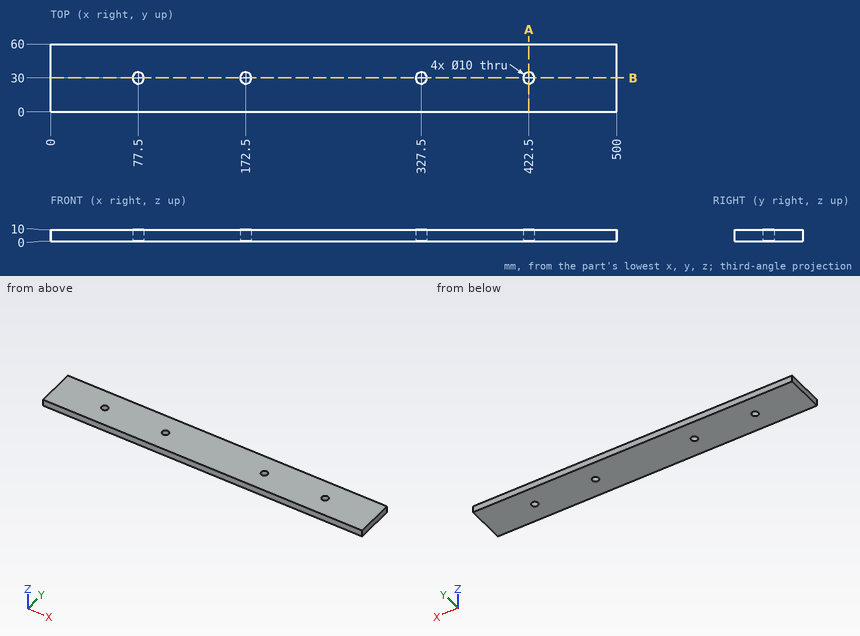
Job drawing, mm, ordinate dimensions from the low corner. One solid piece. Round coordinates to 2 decimals unless told otherwise and drop trailing zeros. Write each loop counter-clockwise with the first axis right and the second up, starting at its lowest first coordinate (ties: lowest second). Pieces come first, ordered by that corner, then holes.
1) Band-saw the part on B-B, the plane y = 30. List the corners of the cut face in (x, z), and give its area (3 significant figures).
2) Drill centre lines: probe 1 along Y at (x, z) = (422.5, 3.25); probe 2 along Y at (x, z) = (330.5, 6.5). Where is each one in solid material? Low to high.
3) Band-saw the part on A-A, the plane x = 422.5. List the corners of the cut face in (y, z).
Ans:
1. outline: (0, 0) - (72.5, 0) - (72.5, 10) - (0, 10) - close; (82.5, 0) - (167.5, 0) - (167.5, 10) - (82.5, 10) - close; (177.5, 0) - (322.5, 0) - (322.5, 10) - (177.5, 10) - close; (332.5, 0) - (417.5, 0) - (417.5, 10) - (332.5, 10) - close; (427.5, 0) - (500, 0) - (500, 10) - (427.5, 10) - close
1. area: 4,600 mm2
2. probe 1: y = 0 to 25, 35 to 60
2. probe 2: y = 0 to 26, 34 to 60
3. outline: (0, 0) - (25, 0) - (25, 10) - (0, 10) - close; (35, 0) - (60, 0) - (60, 10) - (35, 10) - close
